```python
from build123d import *

# Parameters (mm, degrees)
EXTRUDE001_DEPTH = 7
SKETCH011_W      = 9.4
SKETCH011_H      = 1.9
SKETCH011_W_2    = 4.4
SKETCH011_H_2    = 14.3
PAD008_DEPTH     = 2.4
CHAMFER004_SIZE2 = 2
CHAMFER004_SIZE  = 5
CHAMFER005_SIZE2 = 5
CHAMFER005_SIZE  = 1


with BuildPart() as extrude001:
    # Sketch012 (on CopyDatumPlane) → Extrude001 (new body)
    with BuildSketch(Plane.XY.offset(2.4)):
        Polygon((25, 47.7), (30, 47.7), (30, 44.7), (34.3, 44.7), (34.3, 47.7), (38.3, 47.7), (38.3, 39.7), (25, 39.7), align=None)
    extrude(amount=EXTRUDE001_DEPTH)


with BuildPart() as body005:
    # Sketch011 → Pad008 (new body)
    with BuildSketch(Plane.XY):
        with BuildLine():
            Line((-55.3, 0), (-55.3, 69.9))
            Line((-55.3, 69.9), (55.3, 69.9))
            Line((55.3, 69.9), (55.3, 0))
            Line((55.3, 0), (43.3, 0))
            Line((43.3, 0), (43.3, 5.65))
            Line((43.3, 5.65), (39.85, 5.65))
            Line((39.85, 5.65), (39.85, 0))
            Line((39.85, 0), (35.3, 0))
            Line((35.3, 0), (25, 39.7))
            Line((25, 39.7), (25, 47.9))
            ThreePointArc((25, 47.9), (23.242641, 52.142641), (19, 53.9))
            Line((19, 53.9), (-33.3, 53.9))
            ThreePointArc((-33.3, 53.9), (-37.542641, 52.142641), (-39.3, 47.9))
            Line((-39.3, 47.9), (-39.3, 0))
            Line((-39.3, 0), (-44.85, 0))
            Line((-44.85, 0), (-44.85, 5.65))
            Line((-44.85, 5.65), (-50.15, 5.65))
            Line((-50.15, 5.65), (-50.15, 0))
            Line((-50.15, 0), (-55.3, 0))
        make_face()
        with Locations((-44.9, 65.95)):
            Rectangle(SKETCH011_W, SKETCH011_H, mode=Mode.SUBTRACT)
        with Locations((44.9, 65.95)):
            Rectangle(SKETCH011_W, SKETCH011_H, mode=Mode.SUBTRACT)
        with BuildLine():
            Line((-50.3, 54.9), (-50.3, 20))
            ThreePointArc((-50.3, 20), (-47.3, 17), (-44.3, 20))
            Line((-44.3, 20), (-44.3, 54.9))
            ThreePointArc((-44.3, 54.9), (-47.3, 57.9), (-50.3, 54.9))
        make_face(mode=Mode.SUBTRACT)
        with BuildLine():
            Line((40.6, 52.7), (40.6, 20))
            ThreePointArc((40.6, 20), (45.3, 15.3), (50, 20))
            Line((50, 20), (50, 52.7))
            ThreePointArc((50, 52.7), (45.3, 57.4), (40.6, 52.7))
        make_face(mode=Mode.SUBTRACT)
        with Locations((32.2, 51.85)):
            Rectangle(SKETCH011_W_2, SKETCH011_H_2, mode=Mode.SUBTRACT)
    extrude(amount=PAD008_DEPTH)

    # Fusion: union Extrude001
    add(extrude001.part)

    # Chamfer004
    chamfer004_edges = [body005.edges().sort_by_distance(p)[0] for p in [
        (38.3, 43.7, 9.4),
    ]]
    chamfer004_side = body005.faces().sort_by_distance((38.3, 43.7, 5.9))[0]
    chamfer(chamfer004_edges, length=CHAMFER004_SIZE, length2=CHAMFER004_SIZE2, reference=chamfer004_side)

    # Chamfer005
    chamfer005_edges = [body005.edges().sort_by_distance(p)[0] for p in [
        (34.3, 46.2, 9.4),
    ]]
    chamfer005_side = body005.faces().sort_by_distance((30.400323, 43.283871, 9.4))[0]
    chamfer(chamfer005_edges, length=CHAMFER005_SIZE, length2=CHAMFER005_SIZE2, reference=chamfer005_side)


with BuildPart() as body005_1:
    # Body005 placement: moved
    add(body005.part.moved(Location((80, 0, -20))))


solid = body005_1.part
```
Design review of the part built by this model. Coordinates are the model's own, in mm. A direction names the side the tool comes from. Round coordinates to 2 decimals unless told otherwise and drop trailing zeros. Write each loop counter-clockwise with the first axis right and the second up, starting at its lowest first coordinate (ties: lowest second). Pieces come first, ordered by that corner, then holes. Notation, with made-up numbers: (10.5, 63) -> (30.5, 63) arc R24 ccw to (30.5, 77) -> close; hole circle Ø4 at (88, -32). An arc over 180 degrees is marked (long way). Answer in a Markdown table with one row per item.
Q1. To check wall thickness, follow L1, parallel to Y at x = 129.5, z = -18.75; L2, parallel to Y at x = 129, z = -17.75; L3, parallel to Z at x = 46.5, y = 59.5. State the ranges of each line that lie inside material, in increasing order. Write a range as [from, to].
The answers:
| item | result |
|---|---|
| L1 | [0, 17.89], [54.81, 65], [66.9, 69.9] |
| L2 | [0, 17.1], [55.6, 65], [66.9, 69.9] |
| L3 | [-20, -17.6] |
Q2. Clearance check with flat-ended pins moving along their axes: pin 1 Ø2.5 at (x, z) = (33, -19) entering from -Y; pin 2 Ø3 at (x, z) = (78, -14.5) entering from +Y; pin 3 Ø5.5 at (x, z) = (111.5, -13.5) entering from -Y; pin 4 Ø1.6 at (y, z) = (44, -16.5) entering from +X. State where each tip first meets the part, or that it passes through.
The answers:
| item | result |
|---|---|
| pin 1 | y = 5.65 |
| pin 2 | through |
| pin 3 | y = 39.7 |
| pin 4 | x = 118.3 |
Q3. Take a section at D-D, the plane y = 28. State the section outline as (x, z) points.
The answers:
| item | result |
|---|---|
| outline | (24.7, -20) -> (29.7, -20) -> (29.7, -17.6) -> (24.7, -17.6) -> close; (35.7, -20) -> (40.7, -20) -> (40.7, -17.6) -> (35.7, -17.6) -> close; (108.04, -20) -> (120.6, -20) -> (120.6, -17.6) -> (108.04, -17.6) -> close; (130, -20) -> (135.3, -20) -> (135.3, -17.6) -> (130, -17.6) -> close |
Q4. Take a section at C-C, the plane x = 32.7. State the section outline as (y, z) points, then the cut area to 3 significant figures.
The answers:
| item | result |
|---|---|
| outline | (5.65, -20) -> (17, -20) -> (17, -17.6) -> (5.65, -17.6) -> close; (57.9, -20) -> (65, -20) -> (65, -17.6) -> (57.9, -17.6) -> close; (66.9, -20) -> (69.9, -20) -> (69.9, -17.6) -> (66.9, -17.6) -> close |
| area | 51.5 mm² |
Q5. Take a section at A-A, the plane x = 125.3. State the section outline as (y, z) points, then the cut area to 3 significant figures.
The answers:
| item | result |
|---|---|
| outline | (0, -20) -> (15.3, -20) -> (15.3, -17.6) -> (0, -17.6) -> close; (57.4, -20) -> (65, -20) -> (65, -17.6) -> (57.4, -17.6) -> close; (66.9, -20) -> (69.9, -20) -> (69.9, -17.6) -> (66.9, -17.6) -> close |
| area | 62.2 mm² |
Q6. For faces 1 (the face through (105, 44, -15)), 2 (the face through (114.8, 46.2, -13.1)), 3 (the face through (118.3, 44, -17)), list the 3-axis set-ups (+Z, -Z, +X, -X, +Y, -Y) from which the entire face can be reached by the end or side of a thin tool; tool diameter is ignored.
The answers:
| item | result |
|---|---|
| face 1 | +Z, -Z, -Y |
| face 2 | +Z, +Y |
| face 3 | +Z, +X, +Y, -Y |
Q7. Draft analysis for pull direction Y (two halves, no side actions). For faces 4 (the face through (35, 66.9, -19)), 5 (the face through (112, 39.7, -14)), 6 (the face through (111, 43, -10.6)), state which applies: +Y half, -Y half, draft (parallel to the pull), parting line (faces both ways), or undercut.
The answers:
| item | result |
|---|---|
| face 4 | undercut |
| face 5 | -Y half |
| face 6 | draft |
Q8. Take a section at B-B, the plane y = 43. State the section outline as (x, z) points.
The answers:
| item | result |
|---|---|
| outline | (24.7, -20) -> (29.7, -20) -> (29.7, -17.6) -> (24.7, -17.6) -> close; (35.7, -20) -> (40.7, -20) -> (40.7, -17.6) -> (35.7, -17.6) -> close; (105, -20) -> (120.6, -20) -> (120.6, -17.6) -> (118.3, -17.6) -> (118.3, -15.6) -> (116.3, -10.6) -> (105, -10.6) -> close; (130, -20) -> (135.3, -20) -> (135.3, -17.6) -> (130, -17.6) -> close |
